from build123d import *

# Parameters (mm, degrees)
EXTRUDE_1_DEPTH = 3
SKETCH_2_W      = 62
SKETCH_2_H      = 37
EXTRUDE_2_DEPTH = 26


with BuildPart() as part:
    # 草图1 → 凸台-拉伸1 (new body)
    with BuildSketch(Plane.XY):
        with BuildLine():
            Line((0, 0), (62, 0))
            Line((62, 0), (68.5, -16.5))
            Line((68.5, -16.5), (64.5, -16.5))
            ThreePointArc((64.5, -16.5), (62.5, -18.5), (64.5, -20.5))
            Line((64.5, -20.5), (68.5, -20.5))
            Line((68.5, -20.5), (62, -37))
            Line((62, -37), (0, -37))
            Line((0, -37), (-6.5, -20.5))
            Line((-6.5, -20.5), (-2.5, -20.5))
            ThreePointArc((-2.5, -20.5), (-0.5, -18.5), (-2.5, -16.5))
            Line((-2.5, -16.5), (-6.5, -16.5))
            Line((-6.5, -16.5), (0, 0))
        make_face()
    extrude(amount=EXTRUDE_1_DEPTH)

    # 草图2 → 凸台-拉伸2 (add)
    with BuildSketch(Plane.XY.offset(3)):
        with Locations((31, -18.5)):
            Rectangle(SKETCH_2_W, SKETCH_2_H)
    extrude(amount=EXTRUDE_2_DEPTH)


solid = part.part
Verification items for the finished model (mm, model axes). A direction names the side the tool comes from. Round coordinates to 2 decimals unless told otherwise and drop trailing zeros. Loops run counter-clockwise (first coordinate to the right, second up) from the corner with the lowest first, then second, coordinate; pieces in that order, holes last. Notation, with made-up numbers: (33.5, -33.75) - (84.5, -33.75) arc R27 ccw to (84.5, -0.75) - close; hole circle Ø6 at (18, -21). An arc over 180 degrees is marked (long way). Use a Markdown table: item, result. Add a question column.
1. Access from +Z, -Z, +X, -X, +Y, -Y to the whole of each face (thin tool, end or side, straight path). Record for faces 1 (the face through (-4, -16.5, 1)), 2 (the face through (-0.3, -18.2, 3)), 3 (the face through (62, -19, 16)).
2. Section check A-A, the plane x = 63.5. Record the boundary of the cut face in (y, z).
3. Section check D-D, the plane y = -5. Record the boundary of the cut face in (x, z).
4. Section check C-C, the plane z = 4. Record the boundary of the cut face in (x, y).
5. Section check B-B, the plane y = -18.5. Record the boundary of the cut face in (x, z), plus the area to 3 significant figures.
6. Gauge pin test, flat ends, axial feed: pin 1 (8 mm diameter, centred on y = -19, z = 21, fed in from -X); pin 2 (1.5 mm diameter, centred on x = 34.5, z = 9.5, fed in from +Y); pin 3 (3 mm diameter, centred on x = 64, y = -15.5, fed in from +Z). Record the tip position at first contact, or that the pin passes through.
7. Release check for a two-part mould opening along Y. For faces 4 (the face through (31, 0, 14)), 5 (the face through (0, -19, 16)), 6 (the face through (66, -20.5, 1)) record: released by +Y, released by -Y, zero draft, split by the parting line, or undercut.
8. Thickness scan on probe 1 along X at (y, z) = (-18.5, 9.75); probe 2 along Z at (x, y) = (-1, -17). Record the ranges inside material, lowest first. Write a range as [from, to].
Checks:
| question | item | result |
|---|---|---|
| 1 | face 1 | +Z, -Z, -X |
| 1 | face 2 | +Z, -X, +Y, -Y |
| 1 | face 3 | +Z, +X, +Y, -Y |
| 2 | outline | (-33.19, 0) - (-20.23, 0) - (-20.23, 3) - (-33.19, 3) - close; (-16.77, 0) - (-3.81, 0) - (-3.81, 3) - (-16.77, 3) - close |
| 3 | outline | (-1.97, 0) - (63.97, 0) - (63.97, 3) - (62, 3) - (62, 29) - (0, 29) - (0, 3) - (-1.97, 3) - close |
| 4 | outline | (0, -37) - (62, -37) - (62, 0) - (0, 0) - close |
| 5 | outline | (-0.5, 0) - (62.5, 0) - (62.5, 3) - (62, 3) - (62, 29) - (0, 29) - (0, 3) - (-0.5, 3) - close |
| 5 | area | 1,800 mm^2 |
| 6 | pin 1 | stops at x = 0 |
| 6 | pin 2 | stops at y = 0 |
| 6 | pin 3 | stops at z = 3 |
| 7 | face 4 | released by +Y |
| 7 | face 5 | zero draft |
| 7 | face 6 | undercut |
| 8 | probe 1 | x = [0, 62] |
| 8 | probe 2 | z = [0, 3] |
